```python
from build123d import *

# Parameters (mm, degrees)
F0_W     = 15
F0_H     = 9
F1_DEPTH = 4.5
F2_R     = 4.5
F3_DEPTH = 2.5
F4_R     = 1.7
F5_DEPTH = 7.001
F6_SIZE  = 0.5


with BuildPart() as f1:
    # F0 (on Top) → F1 (new body)
    with BuildSketch(Plane.XY):
        Rectangle(F0_W, F0_H)
    extrude(amount=F1_DEPTH)

    # F2 (on face) → F3 (join)
    with BuildSketch(Plane.XY.offset(4.5)):
        Circle(F2_R)
    extrude(amount=F3_DEPTH)

    # F4 (on face) → F5 (cut, through all)
    with BuildSketch(Plane.XY.offset(7)):
        Circle(F4_R)
    extrude(amount=-F5_DEPTH, mode=Mode.SUBTRACT)

    # F6
    f6_edges = [f1.edges().sort_by_distance(p)[0] for p in [
        (-7.5, 0, 4.5),
        (7.5, 0, 4.5),
        (-7.5, -4.5, 2.25),
        (-7.5, 4.5, 2.25),
        (7.5, -4.5, 2.25),
        (7.5, 4.5, 2.25),
        (0, 4.5, 0),
        (7.5, 0, 0),
        (0, -4.5, 0),
        (-7.5, 0, 0),
    ]]
    chamfer(f6_edges, length=F6_SIZE)


solid = f1.part
```
Build history of the part. All positions in model axes, mm. A direction names the side the tool comes from. Round coordinates to 2 decimals unless told otherwise and drop trailing zeros. Order: outer loops, then holes, each group sorted by start corner. A loop starts at its lowest first (then second) coordinate and runs counter-clockwise, first axis right, second up. Notation, with made-up numbers: (73.25, 53) -> (87.25, 53) arc R18 ccw to (87.25, 69) -> close; hole circle Ø7 at (5.25, -24.75). An arc over 180 degrees is marked (long way). Answer in a Markdown table with one row per item.
1) Band-saw the part on B-B on z = 2.5. Give the cut face in (x, y).
Values:
| item | result |
|---|---|
| outline | (-7.5, -4) -> (-7, -4.5) -> (7, -4.5) -> (7.5, -4) -> (7.5, 4) -> (7, 4.5) -> (-7, 4.5) -> (-7.5, 4) -> close; hole circle Ø3.4 at (0, 0) |
2) Mould opens along X. For faces 1 (the cylindrical face through (-0.37, -1.66, 3.55)), 2 (the cylindrical face through (-0.59, 4.46, 5.73)), 3 (the flat face through (7.5, 0, 2)), 4 (the flat face through (0, 2, 0)) say: released by +X, released by -X, zero draft, split by the parting line, or undercut.
Values:
| item | result |
|---|---|
| face 1 | undercut |
| face 2 | split by the parting line |
| face 3 | released by +X |
| face 4 | zero draft |
3) Band-saw the part on C-C on x = 1.25. Give the cut face in (y, z), and give its area (3 significant figures).
Values:
| item | result |
|---|---|
| outline | (-4.5, 0.5) -> (-4, 0) -> (-1.15, 0) -> (-1.15, 7) -> (-4.32, 7) -> (-4.32, 4.5) -> (-4.5, 4.5) -> close; (1.15, 0) -> (4, 0) -> (4.5, 0.5) -> (4.5, 4.5) -> (4.32, 4.5) -> (4.32, 7) -> (1.15, 7) -> close |
| area | 45.7 mm2 |
4) Which spindle directions (+Z, -Z, +X, -X, +Y, -Y) get a long thin tool onto all of the face, cutting with end or side? Do faces 5 (the flat face through (5, 0, 4.5)), 6 (the flat face through (0, -4.5, 2)), 7 (the flat face through (-5, 0, 4.5)). Say none if no direction does.
Values:
| item | result |
|---|---|
| face 5 | +Z, +X |
| face 6 | +Z, -Z, +X, -X, -Y |
| face 7 | +Z, -X |
5) Band-saw the part on D-D on x = -2.5. Give the cut face in (y, z).
Values:
| item | result |
|---|---|
| outline | (-4.5, 0.5) -> (-4, 0) -> (4, 0) -> (4.5, 0.5) -> (4.5, 4.5) -> (3.74, 4.5) -> (3.74, 7) -> (-3.74, 7) -> (-3.74, 4.5) -> (-4.5, 4.5) -> close |
6) Wall check: L1, parallel to Y at x = 0, z = 4.75; L2, parallel to X at y = 0.75, z = 3; L3, parallel to Y at x = 0.5, z = 3.25. Give the ranges that are in metal, low to high.
Values:
| item | result |
|---|---|
| L1 | -4.5 to -1.7, 1.7 to 4.5 |
| L2 | -7.5 to -1.53, 1.53 to 7.5 |
| L3 | -4.5 to -1.62, 1.62 to 4.5 |
7) Pin check, flat tip, straight feed: P1, Ø2, axis at y = -3.5, z = 6, coming from the -X side. Stop position of the tip, or through.
Values:
| item | result |
|---|---|
| P1 | x = -3.74 |
8) Band-saw the part on A-A on y = 0. Give the cut face in (x, z).
Values:
| item | result |
|---|---|
| outline | (-7.5, 0.5) -> (-7, 0) -> (-1.7, 0) -> (-1.7, 7) -> (-4.5, 7) -> (-4.5, 4.5) -> (-7, 4.5) -> (-7.5, 4) -> close; (1.7, 0) -> (7, 0) -> (7.5, 0.5) -> (7.5, 4) -> (7, 4.5) -> (4.5, 4.5) -> (4.5, 7) -> (1.7, 7) -> close |
